Design review of the part built by this model. Coordinates are the model's own, in mm. Face numbers are marked on the shaded views. A direction names the side the tool comes from. Coordinates: 2 decimals unless noted, no trailing zeros. Order: outer loops, then holes, each group sorted by start corner. A loop starts at its lowest first (then second) coordinate and runs counter-clockwise, first axis right, second up. Notation, with made-up numbers: M 73,-27 L 94,-27 A14 cw 94,-5 Z; hole C 3,8.5 d4. An arc over 180 degrees is marked long. Answer as a JSON object with one key per item and string values.
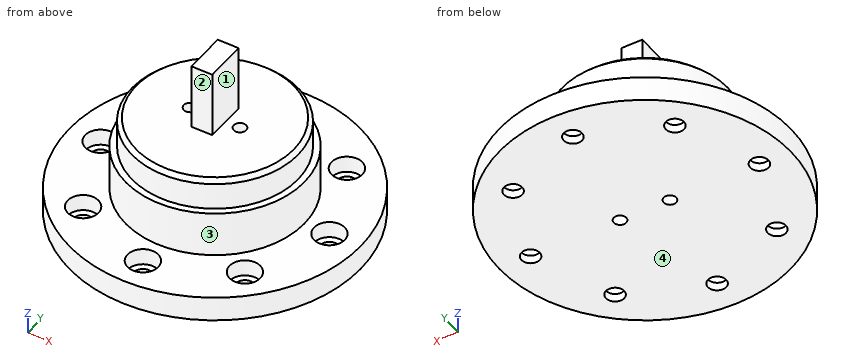
from build123d import *

# Parameters (mm, degrees)
SKETCH1_R           = 35
SKETCH1_R_2         = 2.2
BOSS_EXTRUDE1_DEPTH = 2
SKETCH2_R           = 35
SKETCH2_R_2         = 3.7
BOSS_EXTRUDE2_DEPTH = 4
SKETCH4_R           = 19.95
BOSS_EXTRUDE3_DEPTH = 18.5
SKETCH6_W           = 5
SKETCH6_H           = 10
BOSS_EXTRUDE4_DEPTH = 16
SKETCH7_R           = 21.5
BOSS_EXTRUDE5_DEPTH = 11
SKETCH5_R           = 1.5
CUT_EXTRUDE1_DEPTH  = 25.5
CHAMFER1_SIZE       = 1


with BuildPart() as part:
    # Sketch1 → Boss-Extrude1 (new body)
    with BuildSketch(Plane.XY):
        Circle(SKETCH1_R)
        with Locations((0, 27.5)):
            Circle(SKETCH1_R_2, mode=Mode.SUBTRACT)
        with Locations((19.445436483, 19.445436483)):
            Circle(SKETCH1_R_2, mode=Mode.SUBTRACT)
        with Locations((27.5, 0)):
            Circle(SKETCH1_R_2, mode=Mode.SUBTRACT)
        with Locations((19.445436483, -19.445436483)):
            Circle(SKETCH1_R_2, mode=Mode.SUBTRACT)
        with Locations((0, -27.5)):
            Circle(SKETCH1_R_2, mode=Mode.SUBTRACT)
        with Locations((-19.445436483, -19.445436483)):
            Circle(SKETCH1_R_2, mode=Mode.SUBTRACT)
        with Locations((-27.5, 0)):
            Circle(SKETCH1_R_2, mode=Mode.SUBTRACT)
        with Locations((-19.445436483, 19.445436483)):
            Circle(SKETCH1_R_2, mode=Mode.SUBTRACT)
    extrude(amount=BOSS_EXTRUDE1_DEPTH)

    # Sketch2 → Boss-Extrude2 (add)
    with BuildSketch(Plane.XY.offset(2)):
        Circle(SKETCH2_R)
        with Locations((-27.5, 0)):
            Circle(SKETCH2_R_2, mode=Mode.SUBTRACT)
        with Locations((0, -27.5)):
            Circle(SKETCH2_R_2, mode=Mode.SUBTRACT)
        with Locations((27.5, 0)):
            Circle(SKETCH2_R_2, mode=Mode.SUBTRACT)
        with Locations((0, 27.5)):
            Circle(SKETCH2_R_2, mode=Mode.SUBTRACT)
        with Locations((19.445436483, 19.445436483)):
            Circle(SKETCH2_R_2, mode=Mode.SUBTRACT)
        with Locations((19.445436483, -19.445436483)):
            Circle(SKETCH2_R_2, mode=Mode.SUBTRACT)
        with Locations((-19.445436483, -19.445436483)):
            Circle(SKETCH2_R_2, mode=Mode.SUBTRACT)
        with Locations((-19.445436483, 19.445436483)):
            Circle(SKETCH2_R_2, mode=Mode.SUBTRACT)
    extrude(amount=BOSS_EXTRUDE2_DEPTH)

    # Sketch4 → Boss-Extrude3 (add)
    with BuildSketch(Plane.XY.offset(6)):
        Circle(SKETCH4_R)
    extrude(amount=BOSS_EXTRUDE3_DEPTH)

    # Sketch6 → Boss-Extrude4 (add)
    with BuildSketch(Plane.XY.offset(24.5)):
        Rectangle(SKETCH6_W, SKETCH6_H)
    extrude(amount=BOSS_EXTRUDE4_DEPTH)

    # Sketch7 → Boss-Extrude5 (add)
    with BuildSketch(Plane.XY.offset(6)):
        Circle(SKETCH7_R)
    extrude(amount=BOSS_EXTRUDE5_DEPTH)

    # Sketch5 → Cut-Extrude1 (cut, through all)
    with BuildSketch(Plane.XY.offset(24.5)):
        with Locations((-6, 0)):
            Circle(SKETCH5_R)
        with Locations((6, 0)):
            Circle(SKETCH5_R)
    extrude(amount=-CUT_EXTRUDE1_DEPTH, mode=Mode.SUBTRACT)

    # Chamfer1
    chamfer1_edges = [part.edges().sort_by_distance(p)[0] for p in [
        (-19.95, 0, 24.5),
    ]]
    chamfer(chamfer1_edges, length=CHAMFER1_SIZE)


solid = part.part
1) Add section C-C (z = 21). State the section outline as (x, y) points.
Taken from the geometry:
{"outline": "C 0,0 d39.9; hole C -6,0 d3; hole C 6,0 d3"}
2) Tool access review of the marked faces 1, 2, 3 and 4: name each direction out of +Z, -Z, +X, -X, +Y, -Y from which nothing blocks a thin tool from reaching the whole face with its end or side.
Taken from the geometry:
{"face 1": "+Z, +X, +Y, -Y", "face 2": "+Z, +X, -X, -Y", "face 3": "+Z", "face 4": "-Z, +X, -X, +Y, -Y"}
3) Add section A-A (x = 0). Count the separate pieces of the cut face and the enclosed holes in it, and give its area (3 significant figures).
Taken from the geometry:
{"separate pieces": "3", "enclosed holes": "0", "area": "1,270 mm2"}
4) Add section D-D (x = -27.5). State the section outline as (y, z) points, and give its area (3 significant figures).
Taken from the geometry:
{"outline": "M -21.65,0 L -2.2,0 L -2.2,2 L -3.7,2 L -3.7,6 L -21.65,6 Z; M 2.2,0 L 21.65,0 L 21.65,6 L 3.7,6 L 3.7,2 L 2.2,2 Z", "area": "221 mm2"}
5) To check wall thickness, follow L1, parallel to Y at x = 27.5, z = 3.9; L2, parallel to Y at x = -0.5, z = 12.5; L3, parallel to Z at x = 28, y = -17.5. State the ranges of each line that lie inside material, in increasing order.
Taken from the geometry:
{"L1": "y = -21.65 to -3.7, 3.7 to 21.65", "L2": "y = -21.49 to 21.49", "L3": "z = 0 to 6"}
6) Add section B-B (y = 28.5). State the section outline as (x, z) points, and give its area (3 significant figures).
Taken from the geometry:
{"outline": "M -20.32,0 L -1.96,0 L -1.96,2 L -3.56,2 L -3.56,6 L -20.32,6 Z; M 1.96,0 L 20.32,0 L 20.32,6 L 3.56,6 L 3.56,2 L 1.96,2 Z", "area": "207 mm2"}
7) Insertion check: pin 1 Ø6 at (x, y) = (-28.5, -1) entering from +Z; pin 2 Ø5 at (x, y) = (11.5, -17) entering from +Z; pin 3 Ø1.5 at (x, z) = (-12, 16.5) entering from +Y. Each pin has a flat end and moves straight along its axis. Give the tip position at first contact, or say it passes through.
Taken from the geometry:
{"pin 1": "stops at z = 6", "pin 2": "stops at z = 24.5", "pin 3": "stops at y = 18.32"}
